Verification items for the finished model (mm, model axes). Coordinates: 2 decimals unless noted, no trailing zeros. Loops run counter-clockwise (first coordinate to the right, second up) from the corner with the lowest first, then second, coordinate; pieces in that order, holes last. Notation, with made-up numbers: (12, 50.5) - (27, 50.5) arc R23 ccw to (27, 85.5) - close; hole circle Ø8 at (74.25, 9.5). An arc over 180 degrees is marked (long way). One line per item, written item: value. Start each with the question number.
(1) Section check D-D (z = -53). Record the boundary of the cut face in (x, y), plus the area to 3 significant figures.
(2) Section check A-A (z = 61). Record the boundary of the cut face in (x, y) (3 decimals).
(3) Section check B-B (z = 98). Record the boundary of the cut face in (x, y) (3 decimals).
(4) Section check C-C (x = 80). Record the boundary of the cut face in (y, z), plus the area to 3 significant figures.
(5) Thickness scan on probe 1 along X at (y, z) = (5.5, 32) (3 decimals); probe 2 along Z at (x, y) = (-31.5, 0.5) (3 decimals); probe 3 along X at (y, z) = (3.25, 7). Record the ranges inside material, lowest first. Write a range as [from, to].
(6) Gauge pin test, flat end, axial feed: P1, Ø1.9, axis at y = 2.5, z = -86, coming from the -X side. Record the tip position at first contact, or that the pin passes through.
(7) Draft check along X on faces 1 (the face through (30, 3, 109.13)), 2 (the face through (-82.89, 3.22, -106.96)). Enter one of: +X half, -X half, draft (parallel to the pull), parting line (faces both ways), or undercut.
```python
from build123d import *

# Parameters (mm, degrees)
SKETCH1_W           = 200
SKETCH1_H           = 250
SKETCH1_W_2         = 5.4862609
SKETCH1_H_2         = 76.2
SKETCH1_W_3         = 5.715
SKETCH1_H_3         = 9
SKETCH1_W_4         = 9
SKETCH1_H_4         = 5.715
SKETCH1_W_5         = 15
BOSS_EXTRUDE1_DEPTH = 6.35
FILLET1_R           = 60


with BuildPart() as part:
    # Sketch1 → Boss-Extrude1 (new body)
    with BuildSketch(Plane(origin=(0, 0, 0), x_dir=(1, 0, 0), z_dir=(0, 1, 0))):
        Rectangle(SKETCH1_W, SKETCH1_H)
        with Locations((0, 70.435892683)):
            Rectangle(SKETCH1_W_2, SKETCH1_H_2, mode=Mode.SUBTRACT)
        with Locations((57.8575, -60)):
            Rectangle(SKETCH1_W_3, SKETCH1_H_3, mode=Mode.SUBTRACT)
        with Locations((57.8575, -30)):
            Rectangle(SKETCH1_W_3, SKETCH1_H_3, mode=Mode.SUBTRACT)
        with Locations((0, -87.8575)):
            Rectangle(SKETCH1_W_4, SKETCH1_H_4, mode=Mode.SUBTRACT)
        with Locations((-57.8575, -60)):
            Rectangle(SKETCH1_W_3, SKETCH1_H_3, mode=Mode.SUBTRACT)
        with Locations((-57.8575, -30)):
            Rectangle(SKETCH1_W_3, SKETCH1_H_3, mode=Mode.SUBTRACT)
        with Locations((30, -87.8575)):
            Rectangle(SKETCH1_W_4, SKETCH1_H_4, mode=Mode.SUBTRACT)
        with Locations((-84.5, -45)):
            Rectangle(SKETCH1_W_5, SKETCH1_H_2, mode=Mode.SUBTRACT)
        with Locations((-30, -87.8575)):
            Rectangle(SKETCH1_W_4, SKETCH1_H_4, mode=Mode.SUBTRACT)
        with Locations((30, -106.2725)):
            Rectangle(SKETCH1_W_4, SKETCH1_H_4, mode=Mode.SUBTRACT)
        with Locations((0, -106.2725)):
            Rectangle(SKETCH1_W_4, SKETCH1_H_4, mode=Mode.SUBTRACT)
        with Locations((-30, -106.2725)):
            Rectangle(SKETCH1_W_4, SKETCH1_H_4, mode=Mode.SUBTRACT)
        with Locations((0, -2.1425)):
            Rectangle(SKETCH1_W_4, SKETCH1_H_4, mode=Mode.SUBTRACT)
        with Locations((30, -2.1425)):
            Rectangle(SKETCH1_W_4, SKETCH1_H_4, mode=Mode.SUBTRACT)
        with Locations((30, 16.2725)):
            Rectangle(SKETCH1_W_4, SKETCH1_H_4, mode=Mode.SUBTRACT)
        with Locations((0, 16.2725)):
            Rectangle(SKETCH1_W_4, SKETCH1_H_4, mode=Mode.SUBTRACT)
        with Locations((-30, 16.2725)):
            Rectangle(SKETCH1_W_4, SKETCH1_H_4, mode=Mode.SUBTRACT)
        with Locations((-30, -2.1425)):
            Rectangle(SKETCH1_W_4, SKETCH1_H_4, mode=Mode.SUBTRACT)
        with Locations((84.5, -45)):
            Rectangle(SKETCH1_W_5, SKETCH1_H_2, mode=Mode.SUBTRACT)
        with Locations((57.8575, -75)):
            Rectangle(SKETCH1_W_3, SKETCH1_H_3, mode=Mode.SUBTRACT)
        with Locations((-57.8575, -75)):
            Rectangle(SKETCH1_W_3, SKETCH1_H_3, mode=Mode.SUBTRACT)
        with Locations((57.8575, -15)):
            Rectangle(SKETCH1_W_3, SKETCH1_H_3, mode=Mode.SUBTRACT)
        with Locations((-57.8575, -15)):
            Rectangle(SKETCH1_W_3, SKETCH1_H_3, mode=Mode.SUBTRACT)
        with Locations((34.6075, -97.065)):
            Rectangle(SKETCH1_W_3, SKETCH1_H_3, mode=Mode.SUBTRACT)
        with Locations((-34.6075, -97.065)):
            Rectangle(SKETCH1_W_3, SKETCH1_H_3, mode=Mode.SUBTRACT)
        with Locations((34.6075, 7.065)):
            Rectangle(SKETCH1_W_3, SKETCH1_H_3, mode=Mode.SUBTRACT)
        with Locations((-34.6075, 7.065)):
            Rectangle(SKETCH1_W_3, SKETCH1_H_3, mode=Mode.SUBTRACT)
    extrude(amount=BOSS_EXTRUDE1_DEPTH)

    # Fillet1
    fillet1_edges = [part.edges().sort_by_distance(p)[0] for p in [
        (-100, 3.175, -125),
        (100, 3.175, -125),
    ]]
    fillet(fillet1_edges, radius=FILLET1_R)


solid = part.part
```
Responses:
1. outline: (-100, 0) - (-2.74, 0) - (-2.74, 6.35) - (-100, 6.35) - close; (2.74, 0) - (100, 0) - (100, 6.35) - (2.74, 6.35) - close
1. area: 1,240 mm²
2. outline: (-100, 0) - (-92, 0) - (-92, 6.35) - (-100, 6.35) - close; (-77, 0) - (-60.715, 0) - (-60.715, 6.35) - (-77, 6.35) - close; (-55, 0) - (55, 0) - (55, 6.35) - (-55, 6.35) - close; (60.715, 0) - (77, 0) - (77, 6.35) - (60.715, 6.35) - close; (92, 0) - (100, 0) - (100, 6.35) - (92, 6.35) - close
3. outline: (-100, 0) - (-37.465, 0) - (-37.465, 6.35) - (-100, 6.35) - close; (-31.75, 0) - (31.75, 0) - (31.75, 6.35) - (-31.75, 6.35) - close; (37.465, 0) - (100, 0) - (100, 6.35) - (37.465, 6.35) - close
4. outline: (0, -109.72) - (6.35, -109.72) - (6.35, 6.9) - (0, 6.9) - close; (0, 83.1) - (6.35, 83.1) - (6.35, 125) - (0, 125) - close
4. area: 1,010 mm²
5. probe 1: x = [-100, -92], [-77, -60.715], [-55, 55], [60.715, 77], [92, 100]
5. probe 2: z = [-125, -19.13], [-13.415, -0.715], [5, 85], [90.715, 103.415], [109.13, 125]
5. probe 3: x = [-100, -92], [-77, 77], [92, 100]
6. P1: stops at x = -96.55
7. face 1: undercut
7. face 2: -X half
